Could you check a few things on this model? Use its own coordinates, in mm. Coordinates: 2 decimals unless noted, no trailing zeros. Write each loop counter-clockwise with the first axis right and the second up, starting at its lowest first coordinate (ties: lowest second). Pieces come first, ordered by that corner, then holes.
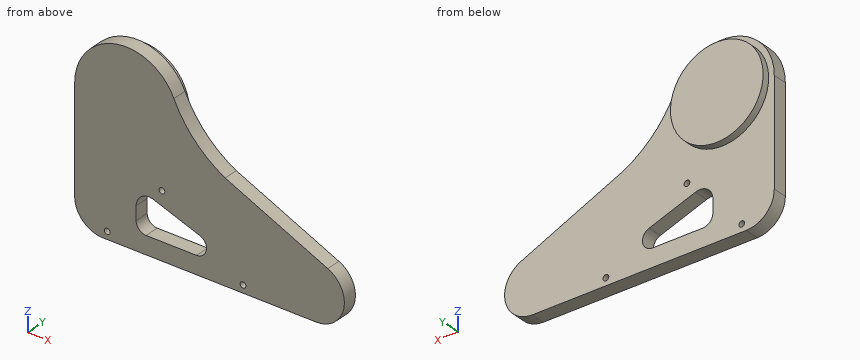
```python
from build123d import *

# Parameters (mm, degrees)
SKETCH2_R           = 2
SKETCH2_R_2         = 32.25
BOSS_EXTRUDE1_DEPTH = 10
SKETCH2_3_R         = 32.25
BOSS_EXTRUDE2_DEPTH = 5


with BuildPart() as part:
    # Sketch2 → Boss-Extrude1 (new body)
    # profile 1 of 2: a face of its own
    with BuildSketch(Plane(origin=(0, 0, 0), x_dir=(1, 0, 0), z_dir=(0, 1, 0))):
        with BuildLine():
            ThreePointArc((-168.164651686, -73), (-139.674052468, -108.34106606), (-99.092179421, -87.998579142))
            ThreePointArc((-99.092179421, -87.998579142), (-84.378455589, -66.061963443), (-63.40890367, -50))
            Line((-63.40890367, -50), (8.019460447, -17.776215731))
            ThreePointArc((8.019460447, -17.776215731), (19.089691145, 3.986136419), (0.23577867, 19.5))
            Line((0.23577867, 19.5), (-148.664651686, 19.5))
            ThreePointArc((-148.664651686, 19.5), (-162.453233919, 13.788582233), (-168.164651686, 0))
            Line((-168.164651686, 0), (-168.164651686, -50))
            Line((-168.164651686, -50), (-168.164651686, -73))
        make_face()
        with Locations(Location((-145.503297495, 14.25, 0), (0, 0, 270))):
            Circle(SKETCH2_R, mode=Mode.SUBTRACT)
        with Locations(Location((-107.4, -25.75, 0), (0, 0, 270))):
            Circle(SKETCH2_R, mode=Mode.SUBTRACT)
        with Locations(Location((-51.003297495, 14.25, 0), (0, 0, 270))):
            Circle(SKETCH2_R, mode=Mode.SUBTRACT)
        with Locations((-132, -73)):
            Circle(SKETCH2_R_2, mode=Mode.SUBTRACT)
        with BuildLine():
            ThreePointArc((-81.121681044, -6.600754354), (-76.542299164, 1.133670887), (-83.352457382, 7))
            Line((-83.352457382, 7), (-118.4, 7))
            ThreePointArc((-118.4, 7), (-123.349747468, 4.949747468), (-125.4, 0))
            Line((-125.4, 0), (-125.4, -9.5))
            ThreePointArc((-125.4, -9.5), (-121.59894333, -16.846494963), (-113.406447056, -17.987557998))
            Line((-113.406447056, -17.987557998), (-81.121681044, -6.600754354))
        make_face(mode=Mode.SUBTRACT)
    # profile 2 of 2: a face of its own
    with BuildSketch(Plane(origin=(0, 0, 0), x_dir=(1, 0, 0), z_dir=(0, 1, 0))):
        with Locations((-132, -73)):
            Circle(SKETCH2_R_2)
    extrude(amount=-BOSS_EXTRUDE1_DEPTH)

    # Sketch2_3 → Boss-Extrude2 (add)
    with BuildSketch(Plane(origin=(0, 0, 0), x_dir=(1, 0, 0), z_dir=(0, 1, 0))):
        with Locations(Location((-132, -73, 0), (0, 0, 270))):
            Circle(SKETCH2_3_R)
    extrude(amount=BOSS_EXTRUDE2_DEPTH)


solid = part.part
```
Item 1: I want a section at D-D, the plane y = -2. List the corners of the cut face in (x, z) for me, then the cut area to 3 significant figures.
Item 2: I want a section at B-B, the plane z = 25.75. List the corners of the cut face in (x, y) for me, then the cut area to 3 significant figures.
Item 3: If I drill on line 1 along X through (y, z) = (-4.25, -14.25); line 2 along X through (y, z) = (-7, -6); line 3 along Z through (x, y) = (-81.5, -6), over which ranges is the centre line in solid material (lowest first)?
Item 4: I want a section at A-A, the plane x = -132. List the corners of the cut face in (y, z) for me, then the cut area to 3 significant figures.
Item 5: I want a section at C-C, the plane x = -86. List the corners of the cut face in (y, z) for me, then the cut area to 3 significant figures.
Item 6: Will these pins go through, and if not, where does the flat tip stop? pin 1 Ø5 at (x, z) = (-145.5, -14.25) entering from +Y; pin 2 Ø1.5 at (x, y) = (-120, -8.5) entering from +Z; pin 3 Ø1 at (x, y) = (-110, -5.5) entering from +Z; pin 4 Ø8 at (y, z) = (-3, -1.5) entering from +X.
Taken from the geometry:
1. outline: (-168.16, 0) arc R19.5 ccw to (-148.66, -19.5) - (0.24, -19.5) arc R19.5 ccw to (8.02, 17.78) - (-63.41, 50) arc R81.3 cw to (-99.09, 88) arc R36.16 ccw to (-168.16, 73) - close; hole circle Ø4 at (-145.5, -14.25); hole (-125.4, 0) arc R7 ccw to (-118.4, -7) - (-83.35, -7) arc R7 ccw to (-81.12, 6.6) - (-113.41, 17.99) arc R9 ccw to (-125.4, 9.5) - close; hole circle Ø4 at (-107.4, 25.75); hole circle Ø4 at (-51, -14.25)
1. area: 14,500 mm2
2. outline: (-168.16, -10) - (-109.4, -10) - (-109.4, 0) - (-168.16, 0) - close; (-105.4, -10) - (-9.66, -10) - (-9.66, 0) - (-105.4, 0) - close
2. area: 1,550 mm2
3. line 1: x = -161.98 to -147.5, -143.5 to -53, -49 to 13.31
3. line 2: x = -167.22 to -122.01, -79.84 to 18.56
3. line 3: z = -19.5 to -6.72, 6.73 to 63.15
4. outline: (-10, -19.5) - (0, -19.5) - (0, 40.75) - (5, 40.75) - (5, 105.25) - (0, 105.25) - (0, 109.16) - (-10, 109.16) - close
4. area: 1,610 mm2
5. outline: (-10, -19.5) - (0, -19.5) - (0, -7) - (-10, -7) - close; (-10, 8.32) - (0, 8.32) - (0, 67.84) - (-10, 67.84) - close
5. area: 720 mm2
6. pin 1: stops at y = 0
6. pin 2: stops at z = 107.37
6. pin 3: stops at z = 102.08
6. pin 4: stops at x = 19.5
